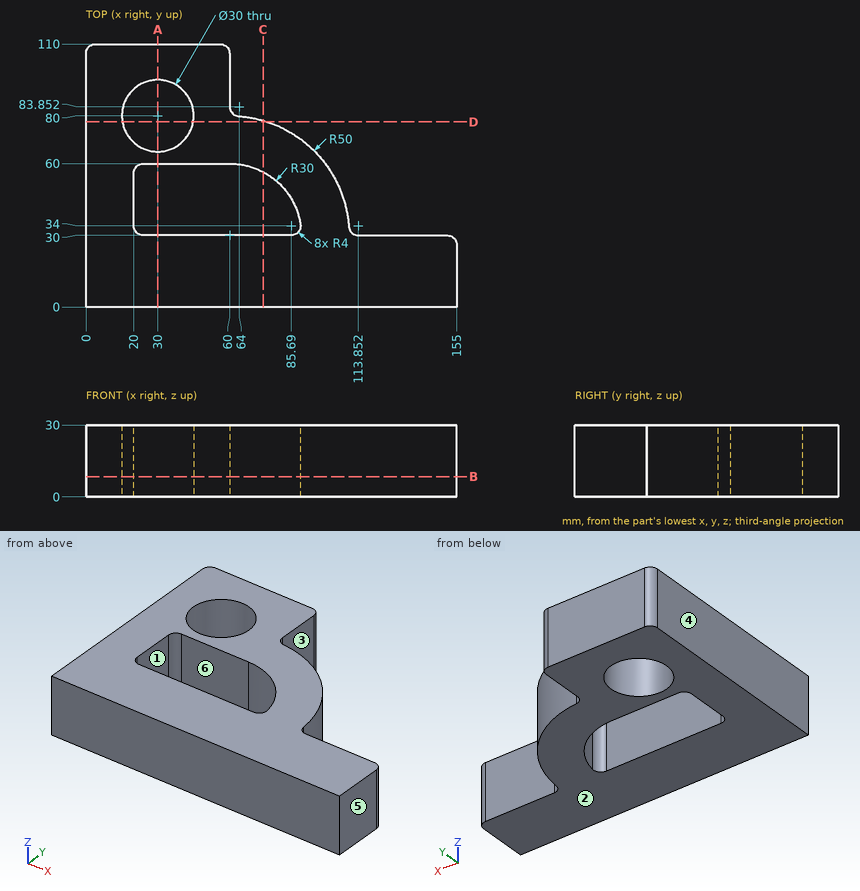
Could you check a few things on this drawing? It's one solid part, dimensions in mm from its lowest x, y, z. A direction names the side the tool comes from. Coordinates: 2 decimals unless noted, no trailing zeros. Order: outer loops, then holes, each group sorted by start corner. A loop starts at its lowest first (then second) coordinate and runs counter-clockwise, first axis right, second up.
1) Will these pins go through, and if not, where does the flat tip stop? pin 1 (9 mm diameter, centred on x = 40, z = 20.5, fed in from -Y); pin 2 (6.5 mm diameter, centred on y = 97, z = 12, fed in from +X); pin 3 (17.5 mm diameter, centred on y = 45, z = 21.5, fed in from +X); pin 4 (12 mm diameter, centred on x = 111, z = 12, fed in from +Y) (1 decimal).
2) Imagine slicing it at B-B on z = 8.5. List the corners of the cut face in (x, y) for me (1 decimal).
3) Imagine slicing it at C-C on x = 74. List the corners of the cut face in (y, z) for me, and give its area (3 significant figures).
4) I need wall thicknesses on line 1 (Y direction, x = 30, z = 6.5); line 2 (Y direction, x = 39, z = 13); line 3 (Y direction, x = 78, z = 16.25). Which ranges of each line are inside material? Lowest first, please.
5) Which directions (+Z, -Z, +X, -X, +Y, -Y) give clear straight access to the entire face, cutting with the end or side of a thin tool? Please do the marked faces 1, 2 and 3.
6) Imagine slicing it at A-A on x = 30. List the corners of the cut face in (y, z) for me.
7) Imagine slicing it at D-D on y = 77.5. List the corners of the cut face in (x, z) for me.
8) We'd pull the mould along X, two halves only. Please class the marked faces 4, 5 and 6: +X half, -X half, draft (parallel to the pull), parting line (faces both ways), or undercut.
Response values:
1. pin 1: stops at y = 0
1. pin 2: stops at x = 60
1. pin 3: stops at x = 109.61
1. pin 4: stops at y = 51.8
2. outline: (0, 0) - (155, 0) - (155, 26) arc R4 ccw to (151, 30) - (113.9, 30) arc R4 cw to (109.9, 33.7) arc R50 ccw to (63.7, 79.9) arc R4 cw to (60, 83.9) - (60, 106) arc R4 ccw to (56, 110) - (4, 110) arc R4 ccw to (0, 106) - close; hole circle Ø30 at (30, 80); hole (20, 34) arc R4 ccw to (24, 30) - (85.7, 30) arc R4 ccw to (89.6, 34.6) arc R30 ccw to (60, 60) - (24, 60) arc R4 ccw to (20, 56) - close
3. outline: (0, 0) - (30, 0) - (30, 30) - (0, 30) - close; (56.53, 0) - (78, 0) - (78, 30) - (56.53, 30) - close
3. area: 1,540 mm2
4. line 1: y = 0 to 30, 60 to 65, 95 to 110
4. line 2: y = 0 to 30, 60 to 68, 92 to 110
4. line 3: y = 0 to 30, 54 to 76.65
5. face 1: +Z, -Z
5. face 2: -Z, +X, -X, +Y, -Y
5. face 3: +Z, -Z, +X, +Y
6. outline: (0, 0) - (30, 0) - (30, 30) - (0, 30) - close; (60, 0) - (65, 0) - (65, 30) - (60, 30) - close; (95, 0) - (110, 0) - (110, 30) - (95, 30) - close
7. outline: (0, 0) - (15.21, 0) - (15.21, 30) - (0, 30) - close; (44.79, 0) - (75.61, 0) - (75.61, 30) - (44.79, 30) - close
8. face 4: -X half
8. face 5: +X half
8. face 6: undercut
